```python
from build123d import *

# Parameters (mm, degrees)
SKETCH1_R      = 4.317999999999999
EXTRUDE1_DEPTH = 2.032
FILLET1_R      = 0.508


with BuildPart() as part:
    # Sketch1 → Extrude1 (new body)
    with BuildSketch(Plane.XY):
        Polygon((-5.125311544677072, 2.9590999999999883), (-6.833748726236091, -2.364e-14), (-5.125311544677051, -2.959100000000024), (-3.4168743631180254, -5.918200000000001), (0, -5.918200000000001), (3.4168743631180534, -5.918200000000001), (5.125311544677072, -2.9590999999999883), (6.833748726236091, 2.45e-14), (5.125311544677051, 2.959100000000024), (3.4168743631180254, 5.918200000000001), (0, 5.918200000000001), (-3.4168743631180534, 5.918200000000001), align=None)
        Circle(SKETCH1_R, mode=Mode.SUBTRACT)
    extrude(amount=EXTRUDE1_DEPTH)

    # Fillet1
    fillet1_edges = [part.edges().sort_by_distance(p)[0] for p in [
        (-5.125311544677058, -2.9591000000000123, 2.032),
        (-1.421e-14, 5.918200000000001, 0),
        (5.125311544677058, 2.9591000000000123, 0),
        (5.125311544677072, -2.959099999999988, 0),
        (1.421e-14, -5.918200000000001, 0),
        (-5.125311544677058, -2.959100000000012, 0),
        (-5.125311544677072, 2.9590999999999883, 0),
        (1.377e-14, -5.918200000000001, 2.032),
        (5.125311544677072, -2.9590999999999883, 2.032),
        (5.125311544677058, 2.9591000000000127, 2.032),
        (-1.377e-14, 5.918200000000001, 2.032),
        (-5.125311544677072, 2.9590999999999887, 2.032),
    ]]
    fillet(fillet1_edges, radius=FILLET1_R)


solid = part.part
```
Read the model definition and answer for the solid it produces. Units are mm, in the model's axes. Give positions to 0.01 mm unless a question says otherwise; leave off trailing zeros. Order: outer loops, then holes, each group sorted by start corner. A loop starts at its lowest first (then second) coordinate and runs counter-clockwise, first axis right, second up. Notation, with made-up numbers: (31, -27) -> (82, -27) arc R30 cw to (82, -5) -> close; hole circle Ø7 at (46.5, -15). An arc over 180 degrees is marked (long way). One line per item, written item: value. Start each with the question number.
(1) The part is cut by section B-B (z = 0.9). Determine the outline of the cut face in (x, y), and give its area (3 significant figures).
(2) The part is cut by section A-A (x = 0). Determine the outline of the cut face in (y, z).
(3) Straight lines are drawn through the part: L1, parallel to Y at x = 0, z = 1.55; L2, parallel to Y at x = -3.5, z = 0.5; L3, parallel to X at y = -3.5, z = 1.2. For each, find the intervals that lie inside material, in ascending order.
(4) The part is cut by section C-C (x = 2.75). Determine the outline of the cut face in (y, z).
(5) For a pull along Y with two mould halves and no side action, classify faces 1 (the cylindrical face through (-4.976, -2.928, 1.879)), 2 (the cylindrical face through (4.976, 2.928, 0.153)), 3 (the cylindrical face through (-0.56, 4.28, 1)) as released by +Y, released by -Y, zero draft, split by the parting line, or undercut.
Taken from the geometry:
1. outline: (-6.83, 0) -> (-3.42, -5.92) -> (3.42, -5.92) -> (6.83, 0) -> (3.42, 5.92) -> (-3.42, 5.92) -> close; hole circle Ø8.64 at (0, 0)
1. area: 62.8 mm^2
2. outline: (-5.92, 0.51) arc R0.51 ccw to (-5.41, 0) -> (-4.32, 0) -> (-4.32, 2.03) -> (-5.41, 2.03) arc R0.51 ccw to (-5.92, 1.52) -> close; (4.32, 0) -> (5.41, 0) arc R0.51 ccw to (5.92, 0.51) -> (5.92, 1.52) arc R0.51 ccw to (5.41, 2.03) -> (4.32, 2.03) -> close
3. L1: -5.92 to -4.32, 4.32 to 5.92
3. L2: -5.77 to -2.53, 2.53 to 5.77
3. L3: -4.81 to -2.53, 2.53 to 4.81
4. outline: (-5.92, 0.51) arc R0.51 ccw to (-5.41, 0) -> (-3.33, 0) -> (-3.33, 2.03) -> (-5.41, 2.03) arc R0.51 ccw to (-5.92, 1.52) -> close; (3.33, 0) -> (5.41, 0) arc R0.51 ccw to (5.92, 0.51) -> (5.92, 1.52) arc R0.51 ccw to (5.41, 2.03) -> (3.33, 2.03) -> close
5. face 1: released by -Y
5. face 2: released by +Y
5. face 3: undercut
